from build123d import *

# Parameters (mm, degrees)
F0_W     = 150
F0_H     = 150
F0_R     = 6
F1_DEPTH = 19.05
F2_R     = 9.75
F3_DEPTH = 3


with BuildPart() as f1:
    # F0 (on Top) → F1 (new body)
    with BuildSketch(Plane.XY):
        with Locations((75, 75)):
            Rectangle(F0_W, F0_H)
        with Locations((25, 25)):
            Circle(F0_R, mode=Mode.SUBTRACT)
        with Locations((125, 25)):
            Circle(F0_R, mode=Mode.SUBTRACT)
        with Locations((25, 125)):
            Circle(F0_R, mode=Mode.SUBTRACT)
        with Locations((125, 125)):
            Circle(F0_R, mode=Mode.SUBTRACT)
    extrude(amount=F1_DEPTH)

    # F2 (on face) → F3 (cut)
    with BuildSketch(Plane.XY.offset(19.05)):
        with Locations((75, 75)):
            Circle(F2_R)
    extrude(amount=-F3_DEPTH, mode=Mode.SUBTRACT)


solid = f1.part
The model under review builds one solid part; all positions refer to its coordinate system, in mm. A direction names the side the tool comes from. Give positions to 0.01 mm unless a question says otherwise; leave off trailing zeros. Loops run counter-clockwise (first coordinate to the right, second up) from the corner with the lowest first, then second, coordinate; pieces in that order, holes last. Notation, with made-up numbers: (26, 84.25) -> (84, 84.25) arc R24 ccw to (84, 119.25) -> close; hole circle Ø11 at (-36, 69.5). An arc over 180 degrees is marked (long way). Answer as a JSON object with one key per item and string values. Group by question number.
Q1. Tool access review of faces 1 (the cylindrical face through (119, 25, 9)), 2 (the cylindrical face through (73.731, 84.667, 17.571)): name each direction out of +Z, -Z, +X, -X, +Y, -Y from which nothing blocks a thin tool from reaching the whole face with its end or side.
Q2. Wall thickness on line 1 along Y through (x, z) = (125, 11); line 2 along Y through (x, z) = (75, 17.8); line 3 along X through (y, z) = (127.5, 7): over which ranges is each line inside the solid? List them lowest first.
Q3. Take a section at D-D (y = 75). Write out the cut boundary in (x, z), plus the area to 3 significant figures.
Q4. Draft analysis for pull direction Y (two halves, no side actions). For faces 3 (the flat face through (74, 150, 9)), 4 (the flat face through (75, 75, 16.05)), 5 (the flat face through (74, 0, 9)), 6 (the flat face through (74, 59, 19.05)), state which applies: pulls with the +Y half, pulls with the -Y half, needs draft (parallel to the pull), parting line crosses it, or undercut.
Q5. Insertion check: pin 1 (9.5 mm diameter, centred on x = 25, y = 25, fed in from +Z). The pin has a flat end and moves straight along its axis. Give the tip position at first contact, or say it passes through.
Q6. Take a section at C-C (z = 8.5). Write out the cut boundary in (x, y).
Q7. Take a section at A-A (x = 125). Write out the cut boundary in (y, z).
Answer below:
{
 "1": {"face 1": "+Z, -Z", "face 2": "+Z"},
 "2": {"line 1": "y = 0 to 19, 31 to 119, 131 to 150", "line 2": "y = 0 to 65.25, 84.75 to 150", "line 3": "x = 0 to 19.55, 30.45 to 119.55, 130.45 to 150"},
 "3": {"outline": "(0, 0) -> (150, 0) -> (150, 19.05) -> (84.75, 19.05) -> (84.75, 16.05) -> (65.25, 16.05) -> (65.25, 19.05) -> (0, 19.05) -> close", "area": "2,800 mm2"},
 "4": {"face 3": "pulls with the +Y half", "face 4": "undercut", "face 5": "pulls with the -Y half", "face 6": "needs draft"},
 "5": {"pin 1": "passes through"},
 "6": {"outline": "(0, 0) -> (150, 0) -> (150, 150) -> (0, 150) -> close; hole circle Ø12 at (25, 25); hole circle Ø12 at (25, 125); hole circle Ø12 at (125, 25); hole circle Ø12 at (125, 125)"},
 "7": {"outline": "(0, 0) -> (19, 0) -> (19, 19.05) -> (0, 19.05) -> close; (31, 0) -> (119, 0) -> (119, 19.05) -> (31, 19.05) -> close; (131, 0) -> (150, 0) -> (150, 19.05) -> (131, 19.05) -> close"}
}
